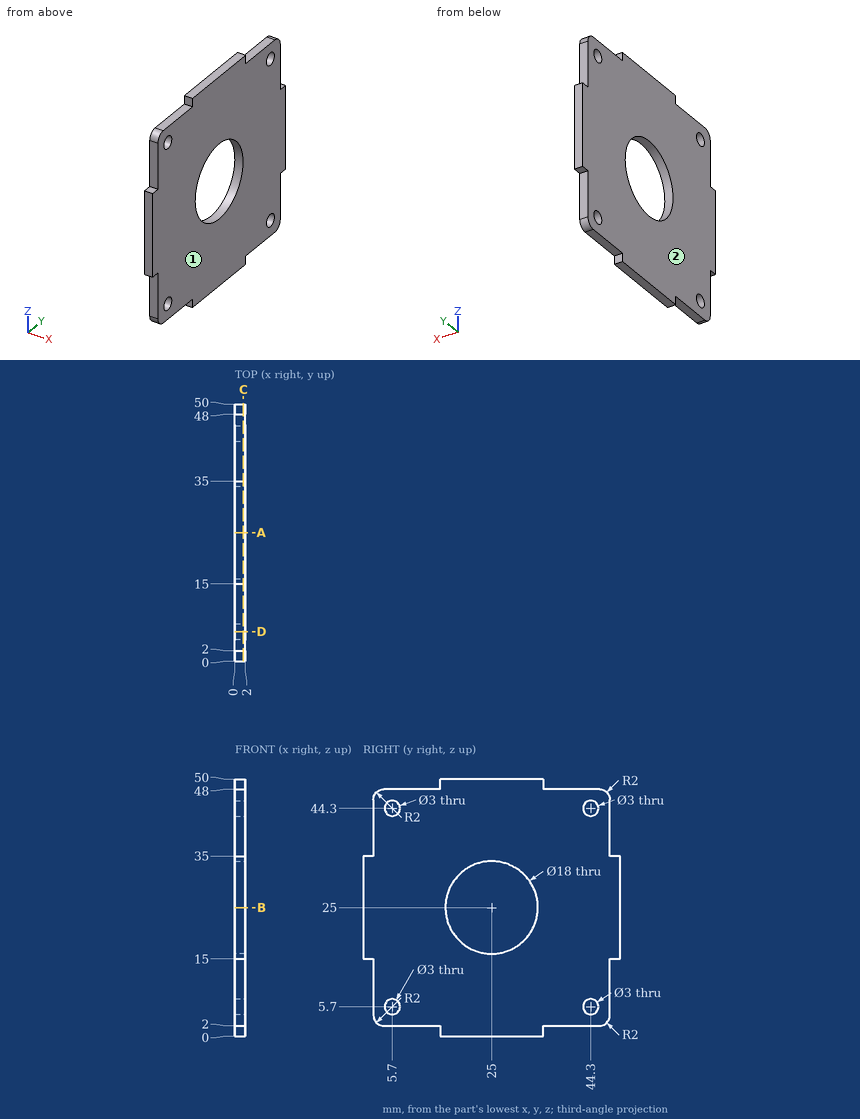
Design review of the part shown in the three views and the two pictorial views. Dimensions are in mm from the part's minimum x, y and z. Round coordinates to 2 decimals unless told otherwise and drop trailing zeros. Loops run counter-clockwise (first coordinate to the right, second up) from the corner with the lowest first, then second, coordinate; pieces in that order, holes last.
Q1. Insertion check: pin 1 Ø0.6 at (x, y) = (1, 48.5) entering from -Z; pin 2 Ø1 at (x, y) = (1, 1) entering from +Z; pin 3 Ø1 at (x, z) = (1.5, 49) entering from +Y. Each pin has a flat end and moves straight along its axis. Give the tip position at first contact, or say it passes through.
Result sheet:
pin 1: stops at z = 15
pin 2: stops at z = 35
pin 3: stops at y = 35
Q2. Add section C-C on x = 1.65. Give the number of separate pieces and of enclosed holes in the cut face, plus the area to 3 significant figures.
Result sheet:
separate pieces: 1
enclosed holes: 5
area: 1,990 mm2
Q3. Mouldability with a two-part tool opening along X and no side actions: class the marked faces 1 and 2 as +X half, -X half, draft (parallel to the pull), parting line (faces both ways), or undercut.
Result sheet:
face 1: +X half
face 2: -X half
Q4. To check wall thickness, follow line 1 along Z through (x, y) = (1.25, 5.7); line 2 along Y through (x, z) = (1, 45). State the ranges of each line that lie inside material, in increasing order.
Result sheet:
line 1: z = 2 to 4.2, 7.2 to 42.8, 45.8 to 48
line 2: y = 2 to 4.37, 7.03 to 42.97, 45.63 to 48
Q5. Add section D-D on y = 5.7. Write out the cut boundary in (x, z), plus the area to 3 significant figures.
Result sheet:
outline: (0, 2) - (2, 2) - (2, 4.2) - (0, 4.2) - close; (0, 7.2) - (2, 7.2) - (2, 42.8) - (0, 42.8) - close; (0, 45.8) - (2, 45.8) - (2, 48) - (0, 48) - close
area: 80.0 mm2
Q6. Add section A-A on y = 25. Write out the cut boundary in (x, z).
Result sheet:
outline: (0, 0) - (2, 0) - (2, 16) - (0, 16) - close; (0, 34) - (2, 34) - (2, 50) - (0, 50) - close
